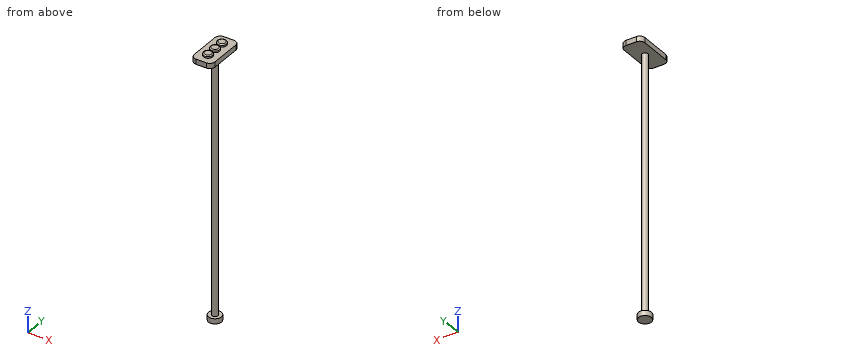
from build123d import *

# Parameters (mm, degrees)
SKETCH2_R                = 5.85
BOSS_EXTRUDE1_DEPTH      = 496
BOSS_EXTRUDE1_DEPTH_BACK = 0.3
SKETCH3_R                = 8.75
BOSS_EXTRUDE2_DEPTH      = 15
FILLET1_R                = 2
BOSS_EXTRUDE3_START      = -25
SKETCH5_R                = 8.75
BOSS_EXTRUDE3_DEPTH      = 15
BOSS_EXTRUDE3_2_DEPTH    = 15
FILLET2_R                = 2
FILLET3_R                = 2
BOSS_EXTRUDE4_START      = -25
BOSS_EXTRUDE4_DEPTH      = 10
SKETCH7_R                = 12.5
BOSS_EXTRUDE5_DEPTH      = 10


with BuildPart() as part:
    # Sketch2 → Boss-Extrude1 (new body, two sides)
    with BuildSketch(Plane.XY) as boss_extrude1_sk:
        Circle(SKETCH2_R)
    extrude(amount=BOSS_EXTRUDE1_DEPTH)
    extrude(boss_extrude1_sk.sketch, amount=-BOSS_EXTRUDE1_DEPTH_BACK)

    # Sketch3 → Boss-Extrude2 (add)
    with BuildSketch(Plane.XY.offset(496)):
        Circle(SKETCH3_R)
    extrude(amount=BOSS_EXTRUDE2_DEPTH)

    # Fillet1
    fillet1_edges = [part.edges().sort_by_distance(p)[0] for p in [
        (-8.75, 0, 511),
    ]]
    fillet(fillet1_edges, radius=FILLET1_R)



with BuildPart() as body_2:
    # Sketch5 → Boss-Extrude3 (new body)
    with BuildSketch(Plane.XY.offset(521).offset(BOSS_EXTRUDE3_START)):
        with Locations((0, 20)):
            Circle(SKETCH5_R)
    extrude(amount=BOSS_EXTRUDE3_DEPTH)

    # Fillet2
    fillet2_edges = [body_2.edges().sort_by_distance(p)[0] for p in [
        (-8.75, 20, 511),
    ]]
    fillet(fillet2_edges, radius=FILLET2_R)


with BuildPart() as body_3:
    # Sketch5 → Boss-Extrude3 2 (new body)
    with BuildSketch(Plane.XY.offset(521).offset(BOSS_EXTRUDE3_START)):
        with Locations((0, -20)):
            Circle(SKETCH5_R)
    extrude(amount=BOSS_EXTRUDE3_2_DEPTH)

    # Fillet3
    fillet3_edges = [body_3.edges().sort_by_distance(p)[0] for p in [
        (-8.75, -20, 511),
    ]]
    fillet(fillet3_edges, radius=FILLET3_R)


with BuildPart() as part_1:
    add(part.part)

    add(body_2.part)  # Boss-Extrude4 merges body 2

    add(body_3.part)  # Boss-Extrude4 merges body 3
    # Sketch6 → Boss-Extrude4 (add)
    with BuildSketch(Plane.XY.offset(521).offset(BOSS_EXTRUDE4_START)):
        with BuildLine():
            Line((10, -40), (-10, -40))
            ThreePointArc((-10, -40), (-17.071067812, -37.071067812), (-20, -30))
            Line((-20, -30), (-20, 30))
            ThreePointArc((-20, 30), (-17.071067812, 37.071067812), (-10, 40))
            Line((-10, 40), (10, 40))
            ThreePointArc((10, 40), (17.071067812, 37.071067812), (20, 30))
            Line((20, 30), (20, -30))
            ThreePointArc((20, -30), (17.071067812, -37.071067812), (10, -40))
        make_face()
    extrude(amount=BOSS_EXTRUDE4_DEPTH)

    # Sketch7 → Boss-Extrude5 (add)
    with BuildSketch(Plane(origin=(0, 0, -0.3), x_dir=(-1, 0, 0), z_dir=(0, 0, -1))):
        Circle(SKETCH7_R)
    extrude(amount=BOSS_EXTRUDE5_DEPTH)


solid = part_1.part
Geometry check sheet. Reference: the model listing, model coordinates, mm. Round coordinates to 2 decimals unless told otherwise and drop trailing zeros. Write each loop counter-clockwise with the first axis right and the second up, starting at its lowest first coordinate (ties: lowest second). Pieces come first, ordered by that corner, then holes. Notation, with made-up numbers: (56, 33) -> (73, 33) arc R26 ccw to (73, 59) -> close; hole circle Ø1 at (20.5, 53). An arc over 180 degrees is marked (long way). One line per item, written item: value. Start each with the question number.
(1) Cross-section at B-B, the plane y = 0. Record the cut outline in (x, z).
(2) Go/stop test with flat-tipped pins: pin 1 Ø2 at (x, y) = (-15, 6) entering from +Z; pin 2 Ø12 at (x, y) = (-5, -19) entering from -Z; pin 3 Ø2 at (y, z) = (8, 310.5) entering from +X. Record where each tip stops, or that it passes through.
(3) Cross-section at D-D, the plane y = -20. Record the cut outline in (x, z).
(4) Scan lines: line 1 (Z direction, x = -13, y = 10); line 2 (Z direction, x = 3, y = -16); line 3 (X direction, y = -5, z = 483). Record each from-to range of solid material in increasing order. Write a range as [from, to].
(5) Cross-section at C-C, the plane z = 93.5. Record the cut outline in (x, y).
Answer:
1. outline: (-20, 496) -> (-5.85, 496) -> (-5.85, -0.3) -> (-12.5, -0.3) -> (-12.5, -10.3) -> (12.5, -10.3) -> (12.5, -0.3) -> (5.85, -0.3) -> (5.85, 496) -> (20, 496) -> (20, 506) -> (8.75, 506) -> (8.75, 509) arc R2 ccw to (6.75, 511) -> (-6.75, 511) arc R2 ccw to (-8.75, 509) -> (-8.75, 506) -> (-20, 506) -> close
2. pin 1: z = 506
2. pin 2: z = 496
2. pin 3: through
3. outline: (-20, 496) -> (20, 496) -> (20, 506) -> (8.75, 506) -> (8.75, 509) arc R2 ccw to (6.75, 511) -> (-6.75, 511) arc R2 ccw to (-8.75, 509) -> (-8.75, 506) -> (-20, 506) -> close
4. line 1: [496, 506]
4. line 2: [496, 511]
4. line 3: [-3.04, 3.04]
5. outline: circle Ø11.7 at (0, 0)
